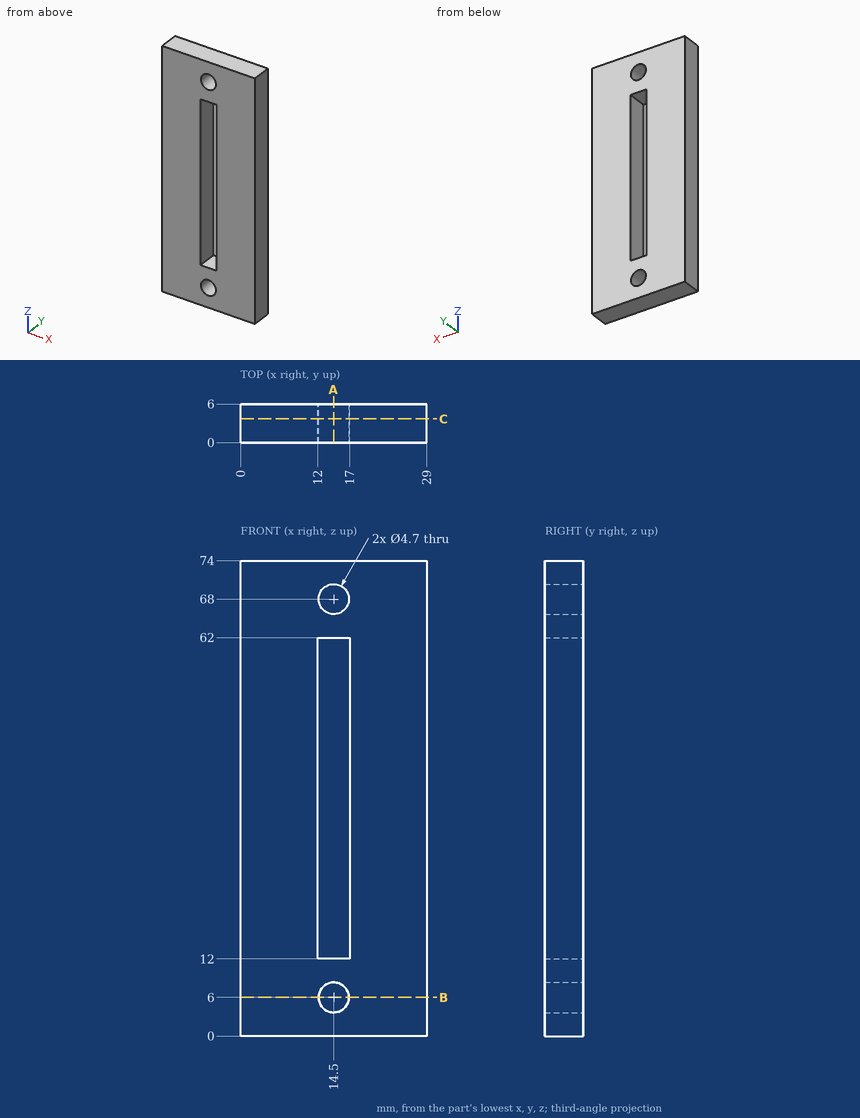
Part print with two shaded views. Sizes in mm from the minimum x, y, z corner. Coordinates: 2 decimals unless noted, no trailing zeros. Write each loop counter-clockwise with the first axis right and the second up, starting at its lowest first coordinate (ties: lowest second). Pieces come first, ordered by that corner, then holes. Notation, with made-up numbers: (69.25, -18) -> (101.25, -18) arc R8 ccw to (101.25, -12) -> close; hole circle Ø8 at (-22.75, 10). An arc over 180 degrees is marked (long way). Return JSON: item names as keys, results as strings. Group by question number.
Q1. Cut at A-A, the plane x = 14.5. Give the cut face in (y, z), then the cut area to 3 significant figures.
Q2. Drill centre lines: line 1 (Z direction, x = 14.5, y = 2.8); line 2 (X direction, y = 1.6, z = 38); line 3 (X direction, y = 4.25, z = 68). Where is each one in solid material? Low to high.
Q3. Cut at B-B, the plane z = 6. Give the cut face in (x, y).
Q4. Cut at C-C, the plane y = 3.7. Give the cut face in (x, z), then the cut area to 3 significant figures.
Returned:
{
 "1": {"outline": "(0, 0) -> (6, 0) -> (6, 3.65) -> (0, 3.65) -> close; (0, 8.35) -> (6, 8.35) -> (6, 12) -> (0, 12) -> close; (0, 62) -> (6, 62) -> (6, 65.65) -> (0, 65.65) -> close; (0, 70.35) -> (6, 70.35) -> (6, 74) -> (0, 74) -> close", "area": "87.6 mm2"},
 "2": {"line 1": "z = 0 to 3.65, 8.35 to 12, 62 to 65.65, 70.35 to 74", "line 2": "x = 0 to 12, 17 to 29", "line 3": "x = 0 to 12.15, 16.85 to 29"},
 "3": {"outline": "(0, 0) -> (12.15, 0) -> (12.15, 6) -> (0, 6) -> close; (16.85, 0) -> (29, 0) -> (29, 6) -> (16.85, 6) -> close"},
 "4": {"outline": "(0, 0) -> (29, 0) -> (29, 74) -> (0, 74) -> close; hole (12, 12) -> (17, 12) -> (17, 62) -> (12, 62) -> close; hole circle Ø4.7 at (14.5, 6); hole circle Ø4.7 at (14.5, 68)", "area": "1,860 mm2"}
}
